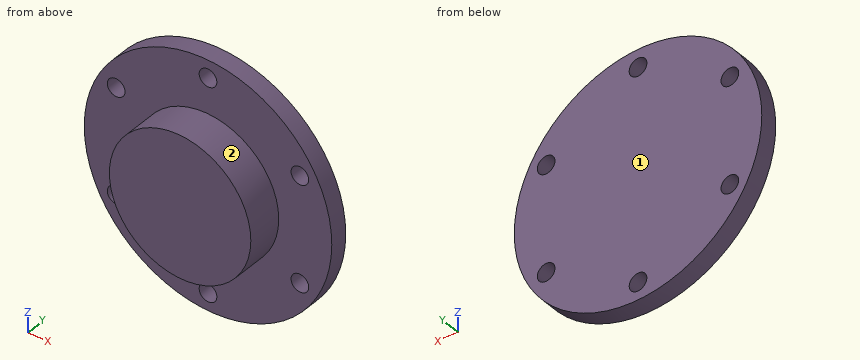
```python
from build123d import *

# Parameters (mm, degrees)
F0_R     = 44.45
F1_DEPTH = 6.35
F2_R     = 25.4
F3_DEPTH = 12.7
F5_R     = 28.575
F5_R_2   = 25.4
F6_DEPTH = 3.175
F7_R     = 3.175
F8_DEPTH = 25.4


with BuildPart() as f1:
    # F0 (on Front) → F1 (new body)
    with BuildSketch(Plane.XZ):
        Circle(F0_R)
    extrude(amount=F1_DEPTH)

    # F2 (on face) → F3 (join)
    with BuildSketch(Plane.XZ.offset(6.35)):
        Circle(F2_R)
    extrude(amount=F3_DEPTH)

    # F5 (on offset) → F6 (cut)
    with BuildSketch(Plane.XZ.offset(12.7)):
        Circle(F5_R)
        Circle(F5_R_2, mode=Mode.SUBTRACT)
    extrude(amount=F6_DEPTH, mode=Mode.SUBTRACT)

    # F7 (on face) → F8 (cut)
    with BuildSketch(Plane(origin=(0, 0, 0), x_dir=(-1, 0, 0), z_dir=(0, 1, 0))):
        with Locations((-32.995568, 19.05)):
            Circle(F7_R)
        with Locations((-32.995568, -19.05)):
            Circle(F7_R)
        with Locations((0, -38.1)):
            Circle(F7_R)
        with Locations((32.995568, -19.05)):
            Circle(F7_R)
        with Locations((32.995568, 19.05)):
            Circle(F7_R)
        with Locations((0, 38.1)):
            Circle(F7_R)
    extrude(amount=-F8_DEPTH, mode=Mode.SUBTRACT)


solid = f1.part
```
Work out the finished part from the listing and answer in its coordinate system (mm). Face numbers are marked on the shaded views. A direction names the side the tool comes from. Give positions to 0.01 mm unless a question says otherwise; leave off trailing zeros. Loops run counter-clockwise (first coordinate to the right, second up) from the corner with the lowest first, then second, coordinate; pieces in that order, holes last. Notation, with made-up numbers: (-22, 74.25) - (-9, 74.25) arc R21 ccw to (-9, 97.25) - close; hole circle Ø9 at (-12.75, 44). An arc over 180 degrees is marked (long way). Use CSV: the item, a comma, the result in double quotes. Start each with the question number.
(1) Find section D-D, the plane x = 22.5. Determine the outline of the cut face in (y, z).
(2) Find the intervals of material crossed by L1, parallel to Z at x = 0, y = -2 (3 decimals); L2, parallel to Z at x = -32, y = -4.25; L3, parallel to Y at x = -31, z = 6, in increasing order.
(3) Find section A-A, the plane x = 35. Determine the outline of the cut face in (y, z), plus the area to 3 significant figures.
(4) A tool of negligible diameter and unlimited length cuts with its end or side. For the marked faces 1 and 2, from which of +Z, -Z, +X, -X, +Y, -Y can it reach the whole face along a straight path? Write none if from no direction.
(5) Find section B-B, the plane z = 0. Determine the outline of the cut face in (x, y).
(6) Find section C-C, the plane z = -19.05. Determine the outline of the cut face in (x, y), plus the area to 3 significant figures.
(7) Each of these flat-tipped pins is pushed along its axis until it touches: pin 1 (10 mm diameter, centred on x = 28, y = -5, fed in from -Z); pin 2 (10 mm diameter, centred on x = 33, z = -19.05, fed in from -Y); pin 3 (6 mm diameter, centred on x = 29.5, y = -6, fed in from -Z); pin 4 (4 mm diameter, centred on x = 34, z = 30.5, fed in from +Y). Where does it stop, or does it pass through?
Results found:
1,outline,"(-19.05, -11.79) - (-6.35, -11.79) - (-6.35, -38.33) - (0, -38.33) - (0, 38.33) - (-6.35, 38.33) - (-6.35, 11.79) - (-19.05, 11.79) - close"
2,L1,"-44.45 to -41.275, -34.925 to 34.925, 41.275 to 44.45"
2,L2,"-30.85 to -22.06, -16.04 to 16.04, 22.06 to 30.85"
2,L3,"-6.35 to 0"
3,outline,"(-6.35, -27.4) - (0, -27.4) - (0, -21.51) - (-6.35, -21.51) - close; (-6.35, -16.59) - (0, -16.59) - (0, 16.59) - (-6.35, 16.59) - close; (-6.35, 21.51) - (0, 21.51) - (0, 27.4) - (-6.35, 27.4) - close"
3,area,"285 mm^2"
4,face 1,"+Z, -Z, +X, -X, +Y"
4,face 2,"-Y"
5,outline,"(-44.45, -6.35) - (-25.4, -6.35) - (-25.4, -19.05) - (25.4, -19.05) - (25.4, -6.35) - (44.45, -6.35) - (44.45, 0) - (-44.45, 0) - close"
6,outline,"(-40.16, -6.35) - (-36.17, -6.35) - (-36.17, 0) - (-40.16, 0) - close; (-29.82, -6.35) - (-16.8, -6.35) - (-16.8, -19.05) - (16.8, -19.05) - (16.8, -6.35) - (29.82, -6.35) - (29.82, 0) - (-29.82, 0) - close; (36.17, -6.35) - (40.16, -6.35) - (40.16, 0) - (36.17, 0) - close"
6,area,"856 mm^2"
7,pin 1,"z = -38.04"
7,pin 2,"y = -6.35"
7,pin 3,"z = -35.69"
7,pin 4,"y = 0"
